from build123d import *

# Parameters (mm, degrees)
BOSS_EXTRUDE1_DEPTH = 4


with BuildPart() as part:
    # Sketch1 → Boss-Extrude1 (new body)
    with BuildSketch(Plane.YZ):
        Polygon((0, 350), (0, 0), (80, 0), (80, 70), (130, 70), (130, 0), (310, 0), (310, 70), (360, 70), (360, 0), (440, 0), (440, 350), align=None)
        with BuildLine():
            Line((7.1, 87.1), (32.9, 87.1))
            ThreePointArc((32.9, 87.1), (35, 85), (32.9, 82.9))
            Line((32.9, 82.9), (7.1, 82.9))
            ThreePointArc((7.1, 82.9), (5, 85), (7.1, 87.1))
        make_face(mode=Mode.SUBTRACT)
        with BuildLine():
            Line((177.9, 7.1), (177.9, 32.9))
            ThreePointArc((177.9, 32.9), (180, 35), (182.1, 32.9))
            Line((182.1, 32.9), (182.1, 7.1))
            ThreePointArc((182.1, 7.1), (180, 5), (177.9, 7.1))
        make_face(mode=Mode.SUBTRACT)
        with BuildLine():
            ThreePointArc((32.9, 157.1), (35, 155), (32.9, 152.9))
            Line((32.9, 152.9), (7.1, 152.9))
            ThreePointArc((7.1, 152.9), (5, 155), (7.1, 157.1))
            Line((7.1, 157.1), (32.9, 157.1))
        make_face(mode=Mode.SUBTRACT)
        with BuildLine():
            ThreePointArc((257.9, 32.9), (260, 35), (262.1, 32.9))
            Line((262.1, 32.9), (262.1, 7.1))
            ThreePointArc((262.1, 7.1), (260, 5), (257.9, 7.1))
            Line((257.9, 7.1), (257.9, 32.9))
        make_face(mode=Mode.SUBTRACT)
        with BuildLine():
            ThreePointArc((407.1, 82.9), (405, 85), (407.1, 87.1))
            Line((407.1, 87.1), (432.9, 87.1))
            ThreePointArc((432.9, 87.1), (435, 85), (432.9, 82.9))
            Line((432.9, 82.9), (407.1, 82.9))
        make_face(mode=Mode.SUBTRACT)
        with BuildLine():
            Line((432.9, 152.9), (407.1, 152.9))
            ThreePointArc((407.1, 152.9), (405, 155), (407.1, 157.1))
            Line((407.1, 157.1), (432.9, 157.1))
            ThreePointArc((432.9, 157.1), (435, 155), (432.9, 152.9))
        make_face(mode=Mode.SUBTRACT)
        with BuildLine():
            Line((7.1, 197.1), (32.9, 197.1))
            ThreePointArc((32.9, 197.1), (35, 195), (32.9, 192.9))
            Line((32.9, 192.9), (7.1, 192.9))
            ThreePointArc((7.1, 192.9), (5, 195), (7.1, 197.1))
        make_face(mode=Mode.SUBTRACT)
        with BuildLine():
            ThreePointArc((32.9, 287.1), (35, 285), (32.9, 282.9))
            Line((32.9, 282.9), (7.1, 282.9))
            ThreePointArc((7.1, 282.9), (5, 285), (7.1, 287.1))
            Line((7.1, 287.1), (32.9, 287.1))
        make_face(mode=Mode.SUBTRACT)
        with BuildLine():
            ThreePointArc((407.1, 192.9), (405, 195), (407.1, 197.1))
            Line((407.1, 197.1), (432.9, 197.1))
            ThreePointArc((432.9, 197.1), (435, 195), (432.9, 192.9))
            Line((432.9, 192.9), (407.1, 192.9))
        make_face(mode=Mode.SUBTRACT)
        with BuildLine():
            Line((432.9, 282.9), (407.1, 282.9))
            ThreePointArc((407.1, 282.9), (405, 285), (407.1, 287.1))
            Line((407.1, 287.1), (432.9, 287.1))
            ThreePointArc((432.9, 287.1), (435, 285), (432.9, 282.9))
        make_face(mode=Mode.SUBTRACT)
    extrude(amount=BOSS_EXTRUDE1_DEPTH)


solid = part.part
Source: CAD feature listing. Evaluate the final solid. Frame: model axes, mm. Round coordinates to 2 decimals unless told otherwise and drop trailing zeros. Loops run counter-clockwise (first coordinate to the right, second up) from the corner with the lowest first, then second, coordinate; pieces in that order, holes last. Notation, with made-up numbers: M 50,7 L 85,7 A26 ccw 85,46 Z; hole C 18,24.25 d10. An arc over 180 degrees is marked long. Return JSON: item names as keys, results as strings. Group by question number.
1. Material intervals for line 1 along Y through (x, z) = (3.4, 51.5); line 2 along Z through (x, y) = (1.7, 318), sorted ascending. Write a range as from..to.
2. Section query A-A on y = 335. Output: boundary loops of the cut face in (x, z), and give its area (3 significant figures).
3. Pin query (flat end, axial travel): pin 1 (1.2 mm diameter, centred on x = 1.5, y = 324.5, fed in from -Z). Return the tip coordinate at first contact, or that it passes through.
4. Section query B-B on x = 0.95. State how many separate pieces and enclosed holes the cut face has, and give its area (3 significant figures).
Checks:
{
 "1": {"line 1": "y = 0..80, 130..310, 360..440", "line 2": "z = 70..350"},
 "2": {"outline": "M 0,70 L 4,70 L 4,350 L 0,350 Z", "area": "1,120 mm²"},
 "3": {"pin 1": "stops at z = 70"},
 "4": {"separate pieces": "1", "enclosed holes": "10", "area": "146,000 mm²"}
}
